from build123d import *

# Parameters (mm, degrees)
BASE_EXTRUDE_DEPTH = 9
SKETCH2_W          = 25
SKETCH2_H          = 5
CUT_EXTRUDE1_DEPTH = 8
CHAMFER1_SIZE      = 1
FILLET1_R          = 5


with BuildPart() as part:
    # Sketch1 → Base-Extrude (new body)
    with BuildSketch(Plane.XY):
        Polygon((7, 0), (7, 5), (0, 5), (0, 70), (7, 70), (7, 75), (290, 75), (290, 0), align=None)
    extrude(amount=BASE_EXTRUDE_DEPTH)

    # Sketch2 → Cut-Extrude1 (cut)
    with BuildSketch(Plane.XY.offset(9)):
        Polygon((281, 75), (290, 66), (290, 75), align=None)
        Polygon((290, 9), (281, 0), (290, 0), align=None)
        with Locations((12.5, 72.5)):
            Rectangle(SKETCH2_W, SKETCH2_H)
        with Locations((12.5, 2.5)):
            Rectangle(SKETCH2_W, SKETCH2_H)
    extrude(amount=-CUT_EXTRUDE1_DEPTH, mode=Mode.SUBTRACT)

    # Chamfer1
    chamfer1_edges = [part.edges().sort_by_distance(p)[0] for p in [
        (0, 37.5, 9),
        (290, 37.5, 9),
    ]]
    chamfer(chamfer1_edges, length=CHAMFER1_SIZE)

    # Fillet1
    fillet1_edges = [part.edges().sort_by_distance(p)[0] for p in [
        (7, 5, 0.5),
        (25, 5, 5),
        (7, 70, 0.5),
        (25, 70, 5),
    ]]
    fillet(fillet1_edges, radius=FILLET1_R - 0.0001)  # a hair under: the kernel refuses the full size


solid = part.part
Build history of the part. All positions in model axes, mm. A direction names the side the tool comes from. Round coordinates to 2 decimals unless told otherwise and drop trailing zeros. Use CSV: the item, a comma, the result in double quotes. Start each with the question number.
(1) Tool access for faces 1 (the face through (10, 5, 4)), 2 (the face through (23, 71, 5)), 3 (the face through (287, 73, 1)): list every direction of +Z, -Z, +X, -X, +Y, -Y with a clear straight run to the whole face (end or side of a thin tool).
(2) Flat gauge pins, fed straight in: P1, Ø2.5, axis at x = 18.5, y = 2, coming from the +Z side; P2, Ø5, axis at x = 34.5, y = 17.5, coming from the -Z side; P3, Ø2.5, axis at x = 10, z = 6.5, coming from the +Y side. Where does each tip first touch, or does it go through?
(3) Drill centre lines: probe 1 along Y at (x, z) = (18, 5.75); probe 2 along X at (y, z) = (3.5, 7.25). Where is each one in solid material? Low to high.
Findings:
1,face 1,"+Z, -X, -Y"
1,face 2,"+Z, -X, +Y"
1,face 3,"+Z, +X, +Y"
2,P1,"stops at z = 1"
2,P2,"stops at z = 0"
2,P3,"stops at y = 70"
3,probe 1,"y = 5 to 70"
3,probe 2,"x = 23.57 to 284.5"
